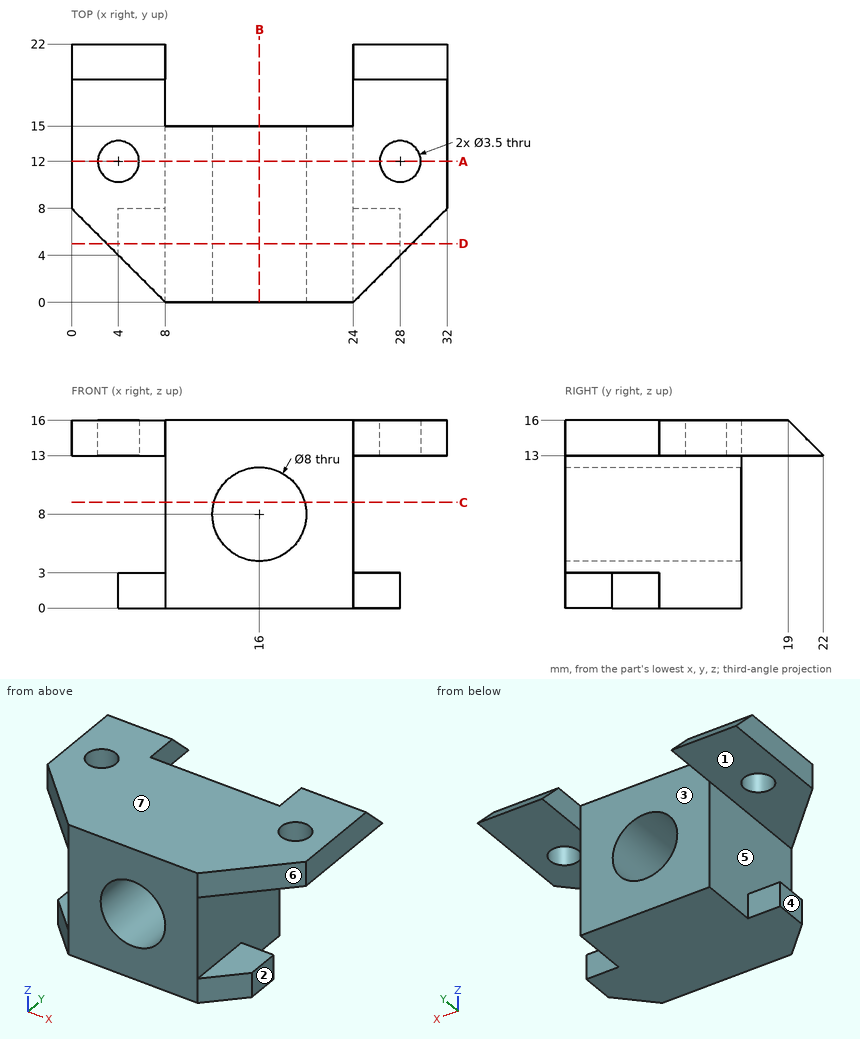
Could you check a few things on this drawing? It's one solid part, dimensions in mm from its lowest x, y, z. A direction names the side the tool comes from. Coordinates: 2 decimals unless noted, no trailing zeros. Order: outer loops, then holes, each group sorted by start corner. A loop starts at its lowest first (then second) coordinate and runs counter-clockwise, first axis right, second up. Notation, with made-up numbers: (-12.75, -30) - (40.25, -30) arc R9 ccw to (40.25, -20) - close; hole circle Ø9 at (-1.75, -35). An arc over 180 degrees is marked (long way). Answer as a JSON object with one key per item and string values. Group by question number.
Q1. Imagine slicing it at B-B (x = 16). Please give me the cut outline in (y, z), and give its area (3 significant figures).
Q2. I need wall thicknesses on line 1 (Y direction, x = 11, z = 15.25); line 2 (X direction, y = 10, z = 8); line 3 (X direction, y = 9.5, z = 1.5). Which ranges of each line are inside material? Lowest first, please. Write a range as from..to.
Q3. Will these pins go through, and if not, where does the flat tip stop? P1, Ø6.5, axis at y = 4, z = 3.5, coming from the -X side; P2, Ø5, axis at y = 7.5, z = 4, coming from the +X side; P3, Ø1.5, axis at x = 26, z = 1.5, coming from the +Y side.
Q4. Imagine slicing it at D-D (y = 5). Please give me the cut outline in (x, z), and give its area (3 significant figures).
Q5. On a 3-axis mill with a long thin cutter (end or side, diameter ignored), from which of +Z, -Z, +X, -X, +Y, -Y can I reach the whole of each face in a straight line? I mean the marked faces 1, 2, 3 and 4. Say none if no direction works.
Q6. Imagine slicing it at C-C (z = 9). Please give me the cut outline in (x, y), and give its area (3 significant figures).
Q7. Imagine slicing it at A-A (y = 12). Please give me the cut outline in (x, z).
Q8. We'd pull the mould along Z, two halves only. Please class the marked faces 5, 6 and 7: +Z half, -Z half, draft (parallel to the pull), parting line (faces both ways), or undercut.
Determined:
{
 "1": {"outline": "(0, 0) - (15, 0) - (15, 4) - (0, 4) - close; (0, 12) - (15, 12) - (15, 16) - (0, 16) - close", "area": "120 mm2"},
 "2": {"line 1": "y = 0..15", "line 2": "x = 8..12, 20..24", "line 3": "x = 8..24"},
 "3": {"P1": "stops at x = 4", "P2": "stops at x = 28", "P3": "stops at y = 8"},
 "4": {"outline": "(3, 13) - (8, 13) - (8, 3) - (4, 3) - (4, 0) - (28, 0) - (28, 3) - (24, 3) - (24, 13) - (29, 13) - (29, 16) - (3, 16) - close; hole circle Ø8 at (16, 8)", "area": "260 mm2"},
 "5": {"face 1": "-X, +Y, -Y", "face 2": "-Z, +X, +Y, -Y", "face 3": "+Z, -Z, +Y", "face 4": "-Z, -X, +Y, -Y"},
 "6": {"outline": "(8, 0) - (12.13, 0) - (12.13, 15) - (8, 15) - close; (19.87, 0) - (24, 0) - (24, 15) - (19.87, 15) - close", "area": "124 mm2"},
 "7": {"outline": "(0, 13) - (2.25, 13) - (2.25, 16) - (0, 16) - close; (5.75, 13) - (8, 13) - (8, 0) - (24, 0) - (24, 13) - (26.25, 13) - (26.25, 16) - (5.75, 16) - close; (29.75, 13) - (32, 13) - (32, 16) - (29.75, 16) - close; hole circle Ø8 at (16, 8)"},
 "8": {"face 5": "undercut", "face 6": "draft", "face 7": "+Z half"}
}
